```python
from build123d import *

# Parameters (mm, degrees)
BOSS_EXTRU_1_DEPTH      = 2
D_GAGEMENT_M3_51_D      = 3.9
ENL_V_MAT_EXTRU_3_DEPTH = 1
D_GAGEMENT_M3_52_D      = 3.9
D_GAGEMENT_M61_D        = 6.6


with BuildPart() as part:
    # Esquisse1 → Boss.-Extru.1 (new body)
    with BuildSketch(Plane.XY):
        with BuildLine():
            ThreePointArc((30, 0), (15, -15), (0, 0))
            Line((0, 0), (0, 70))
            ThreePointArc((0, 70), (15, 85), (30, 70))
            Line((30, 70), (30, 0))
        make_face()
    extrude(amount=BOSS_EXTRU_1_DEPTH)

    # Dégagement M3.51 (through all)
    with Locations(Plane(origin=(0, 0, 0), x_dir=(-1, 0, 0), z_dir=(0, 0, -1))):
        with Locations((-15, 79), (-15, 35)):
            Hole(D_GAGEMENT_M3_51_D / 2)

    # Esquisse5 → Enlèv. mat.-Extru.3 (cut)
    with BuildSketch(Plane(origin=(0, 0, 0), x_dir=(-1, 0, 0), z_dir=(0, 0, -1))):
        Polygon((-12.5, 54.5), (-2.5, 54.5), (-2.5, 59.5), (-12.5, 59.5), (-12.5, 69.5), (-17.5, 69.5), (-17.5, 59.5), (-27.5, 59.5), (-27.5, 54.5), (-17.5, 54.5), (-17.5, 44.5), (-12.5, 44.5), align=None)
    extrude(amount=-ENL_V_MAT_EXTRU_3_DEPTH, mode=Mode.SUBTRACT)

    # Dégagement M3.52 (through all)
    with Locations(Plane(origin=(0, 0, 0), x_dir=(-1, 0, 0), z_dir=(0, 0, -1))):
        with Locations((-15, 0)):
            Hole(D_GAGEMENT_M3_52_D / 2)

    # Dégagement M61 (through all)
    with Locations(Plane(origin=(0, 0, 0), x_dir=(-1, 0, 0), z_dir=(0, 0, -1))):
        with Locations((-15, 57)):
            Hole(D_GAGEMENT_M61_D / 2)


solid = part.part
```
Can you work these out from the model? Positions are in its coordinate system, mm. Coordinates: 2 decimals unless noted, no trailing zeros. Order: outer loops, then holes, each group sorted by start corner. A loop starts at its lowest first (then second) coordinate and runs counter-clockwise, first axis right, second up. Notation, with made-up numbers: (48, 6.25) - (82, 6.25) arc R20 ccw to (82, 20.25) - close; hole circle Ø7 at (-17, 33.5). An arc over 180 degrees is marked (long way). Answer in a Markdown table with one row per item.
1. If I drill on line 1 along Y through (x, z) = (15, 1.4); line 2 along Y through (x, z) = (15, 0.65); line 3 along X through (y, z) = (66, 0.9), over which ranges is the centre line in solid material (lowest first)?
Reply:
| item | result |
|---|---|
| line 1 | y = -15 to -1.95, 1.95 to 33.05, 36.95 to 53.7, 60.3 to 77.05, 80.95 to 85 |
| line 2 | y = -15 to -1.95, 1.95 to 33.05, 36.95 to 44.5, 69.5 to 77.05, 80.95 to 85 |
| line 3 | x = 0 to 12.5, 17.5 to 30 |
2. Suppose I cut it at D-D (y = 35). Please give me the cut outline in (x, z).
Reply:
| item | result |
|---|---|
| outline | (0, 0) - (13.05, 0) - (13.05, 2) - (0, 2) - close; (16.95, 0) - (30, 0) - (30, 2) - (16.95, 2) - close |
3. Suppose I cut it at A-A (y = 57). Please give me the cut outline in (x, z).
Reply:
| item | result |
|---|---|
| outline | (0, 0) - (2.5, 0) - (2.5, 1) - (11.7, 1) - (11.7, 2) - (0, 2) - close; (18.3, 1) - (27.5, 1) - (27.5, 0) - (30, 0) - (30, 2) - (18.3, 2) - close |
4. If we mould it in two halves opening along Y, with no side actions, what happens to faces 1 (the cylindrical face through (15, -15, 1)), 2 (the cylindrical face through (13.453, 33.813, 1.014)), 3 (the flat face through (0, 35, 1)), 4 (the cylindrical face through (13.563, 80.318, 1.014))? For each: pulls with the +Y half, pulls with the -Y half, needs draft (parallel to the pull), parting line crosses it, or undercut.
Reply:
| item | result |
|---|---|
| face 1 | pulls with the -Y half |
| face 2 | undercut |
| face 3 | needs draft |
| face 4 | undercut |
5. Suppose I cut it at C-C (x = 14.75). Please give me the cut outline in (y, z).
Reply:
| item | result |
|---|---|
| outline | (-15, 0) - (-1.93, 0) - (-1.93, 2) - (-15, 2) - close; (1.93, 0) - (33.07, 0) - (33.07, 2) - (1.93, 2) - close; (36.93, 0) - (44.5, 0) - (44.5, 1) - (53.71, 1) - (53.71, 2) - (36.93, 2) - close; (60.29, 1) - (69.5, 1) - (69.5, 0) - (77.07, 0) - (77.07, 2) - (60.29, 2) - close; (80.93, 0) - (85, 0) - (85, 2) - (80.93, 2) - close |
6. For pin 1 (0.8 mm diameter, centred on x = 16, z = 0.5, fed in from -Y); pin 2 (0.5 mm diameter, centred on x = 6, z = 0.5, fed in from -Y); pin 3 (0.5 mm diameter, centred on x = 6, z = 0.5, fed in from +Y), each with a flat end and sliding along its axis, tell me the tip position at first contact or that it passes through.
Reply:
| item | result |
|---|---|
| pin 1 | stops at y = -14.99 |
| pin 2 | stops at y = -12.18 |
| pin 3 | stops at y = 82.18 |
7. Suppose I cut it at B-B (z = 1.3). Please give me the cut outline in (x, y).
Reply:
| item | result |
|---|---|
| outline | (0, 0) arc R15 ccw to (30, 0) - (30, 70) arc R15 ccw to (0, 70) - close; hole circle Ø6.6 at (15, 57); hole circle Ø3.9 at (15, 0); hole circle Ø3.9 at (15, 35); hole circle Ø3.9 at (15, 79) |
